from build123d import *

# Parameters (mm, degrees)
SKETCH_1_R          = 1.1
SKETCH_1_R_2        = 1.6
EXTRUDE_1_DEPTH     = 4
SKETCH_2_W          = 4
SKETCH_2_H          = 6
EXTRUDE_2_DEPTH     = 36
SKETCH_3_R          = 1.6
EXTRUDE_3_DEPTH     = 4
SKETCH_4_W          = 26
SKETCH_4_H          = 5
EXTRUDE_4_DEPTH     = 6
SKETCH_7_R          = 1.1
CUT_EXTRUDE_2_DEPTH = 66.61562314


with BuildPart() as part:
    # ｽｹｯﾁ1 → ﾎﾞｽ - 押し出し1 (new body)
    with BuildSketch(Plane.XY):
        with BuildLine():
            Line((-17, -17), (-17, -23))
            Line((-17, -23), (17, -23))
            Line((17, -23), (17, -17))
            Line((17, -17), (11, -17))
            ThreePointArc((11, -17), (8.878679656, -16.121320344), (8, -14))
            Line((8, -14), (8, 0))
            ThreePointArc((8, 0), (0, 8), (-8, 0))
            Line((-8, 0), (-8, -14))
            ThreePointArc((-8, -14), (-8.878679656, -16.121320344), (-11, -17))
            Line((-11, -17), (-17, -17))
        make_face()
        with Locations((0, 6)):
            Circle(SKETCH_1_R, mode=Mode.SUBTRACT)
        with Locations((4.242640687, 4.242640687)):
            Circle(SKETCH_1_R, mode=Mode.SUBTRACT)
        with Locations((6, 0)):
            Circle(SKETCH_1_R, mode=Mode.SUBTRACT)
        with Locations((4.242640687, -4.242640687)):
            Circle(SKETCH_1_R, mode=Mode.SUBTRACT)
        with Locations((0, -6)):
            Circle(SKETCH_1_R, mode=Mode.SUBTRACT)
        with Locations((-4.242640687, -4.242640687)):
            Circle(SKETCH_1_R, mode=Mode.SUBTRACT)
        with Locations((-6, 0)):
            Circle(SKETCH_1_R, mode=Mode.SUBTRACT)
        with Locations((-4.242640687, 4.242640687)):
            Circle(SKETCH_1_R, mode=Mode.SUBTRACT)
        Circle(SKETCH_1_R_2, mode=Mode.SUBTRACT)
    extrude(amount=EXTRUDE_1_DEPTH)

    # ｽｹｯﾁ2 → ﾎﾞｽ - 押し出し2 (add)
    with BuildSketch(Plane.XY.offset(4)):
        with Locations((-15, -20)):
            Rectangle(SKETCH_2_W, SKETCH_2_H)
        with Locations((15, -20)):
            Rectangle(SKETCH_2_W, SKETCH_2_H)
    extrude(amount=EXTRUDE_2_DEPTH)

    # ｽｹｯﾁ3 → ﾎﾞｽ - 押し出し3 (add)
    with BuildSketch(Plane.XY.offset(40)):
        with BuildLine():
            Line((-11, -17), (-17, -17))
            Line((-17, -17), (-17, -23))
            Line((-17, -23), (17, -23))
            Line((17, -23), (17, -17))
            Line((17, -17), (11, -17))
            ThreePointArc((11, -17), (8.878679656, -16.121320344), (8, -14))
            Line((8, -14), (8, 0))
            ThreePointArc((8, 0), (0, 8), (-8, 0))
            Line((-8, 0), (-8, -14))
            ThreePointArc((-8, -14), (-8.878679656, -16.121320344), (-11, -17))
        make_face()
        Circle(SKETCH_3_R, mode=Mode.SUBTRACT)
    extrude(amount=EXTRUDE_3_DEPTH)

    # ｽｹｯﾁ4 → ﾎﾞｽ - 押し出し4 (add)
    with BuildSketch(Plane(origin=(0, -17, 0), x_dir=(1, 0, 0), z_dir=(0, 1, 0))):
        with Locations((0, -6.5)):
            Rectangle(SKETCH_4_W, SKETCH_4_H)
        with Locations((0, -37.5)):
            Rectangle(SKETCH_4_W, SKETCH_4_H)
    extrude(amount=-EXTRUDE_4_DEPTH)

    # ｽｹｯﾁ7 → ｶｯﾄ - 押し出し2 (cut, through all)
    with BuildSketch(Plane(origin=(-25.9, 0, 44), x_dir=(-1, 0, 0), z_dir=(0, 0, -1))):
        with Locations((-36.4, -20)):
            Circle(SKETCH_7_R)
        with Locations(Location((-15.4, -20, 0), (0, 0, 180))):
            Circle(SKETCH_7_R)
    extrude(amount=CUT_EXTRUDE_2_DEPTH, mode=Mode.SUBTRACT)


solid = part.part
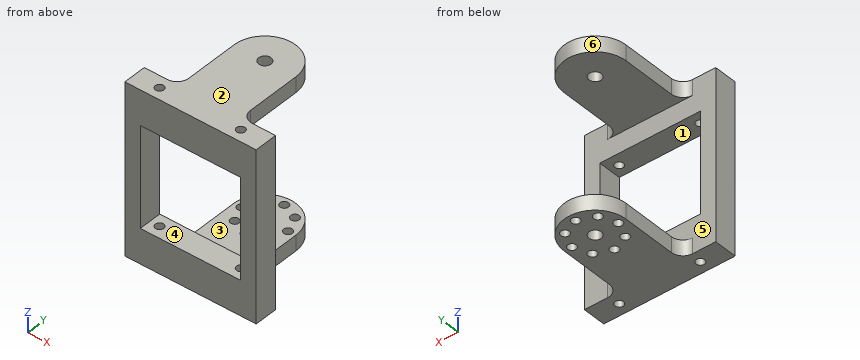
Check sheet for the modelled part. Datum: model origin and axes. Units: mm. Face numbers are marked on the shaded views. A direction names the side the tool comes from. Give positions to 0.01 mm unless a question says otherwise; leave off trailing zeros. Write each loop counter-clockwise with the first axis right and the second up, starting at its lowest first coordinate (ties: lowest second). Pieces come first, ordered by that corner, then holes. Notation, with made-up numbers: (-6.75, 49.25) -> (38.25, 49.25) arc R13 cw to (38.25, 66.25) -> close; hole circle Ø2 at (23.25, 87.5). An arc over 180 degrees is marked (long way). Write item = value, one per line.
Item 1: Sectioned sample at A-A on x = 0. Record the boundary of the cut face in (y, z).
Output:
outline = (-23, 0) -> (-7.1, 0) -> (-7.1, 4) -> (-17, 4) -> (-17, 9) -> (-23, 9) -> close; (-23, 35) -> (-17, 35) -> (-17, 40) -> (-1.6, 40) -> (-1.6, 44) -> (-23, 44) -> close; (-4.9, 0) -> (-1.6, 0) -> (-1.6, 4) -> (-4.9, 4) -> close; (1.6, 0) -> (4.9, 0) -> (4.9, 4) -> (1.6, 4) -> close; (1.6, 40) -> (8, 40) -> (8, 44) -> (1.6, 44) -> close; (7.1, 0) -> (8, 0) -> (8, 4) -> (7.1, 4) -> close
Item 2: Scan lines: probe 1 along Y at (x, z) = (0, 2.2); probe 2 along Z at (x, y) = (-6, 3); probe 3 along Z at (x, y) = (3.5, -21). Record each from-to range of solid material in increasing order. Write a range as from..to.
Output:
probe_1 = -23..-7.1, -4.9..-1.6, 1.6..4.9, 7.1..8
probe_2 = 0..4, 40..44
probe_3 = 0..9, 35..44
Item 3: Gauge pin test, flat ends, axial feed: pin 1 (10 mm diameter, centred on x = 1, z = 13.5, fed in from +Y); pin 2 (4.5 mm diameter, centred on y = -4.5, z = 42, fed in from -X). Record the tip position at first contact, or that the pin passes through.
Output:
pin_1 = -17
pin_2 = -8
Item 4: Tool access check on the marked faces 1, 2 and 3. Record the directions out of +Z, -Z, +X, -X, +Y, -Y that give a thin tool (end or side, any length) a straight path to the whole face; none if there is none.
Output:
face_1 = +Y, -Y
face_2 = +Z, +X, -X, +Y, -Y
face_3 = +X, -X, +Y
Item 5: Release check for a two-part mould opening along X. For the marked faces 4, 5 and 6 record: +X half, -X half, draft (parallel to the pull), parting line (faces both ways), or undercut.
Output:
face_4 = undercut
face_5 = draft
face_6 = parting line
Item 6: Sectioned sample at B-B on y = -20. Record the boundary of the cut face in (x, z), and give its area (3 significant figures).
Output:
outline = (-17, 0) -> (-11.6, 0) -> (-11.6, 9) -> (-13, 9) -> (-13, 35) -> (-11.6, 35) -> (-11.6, 44) -> (-17, 44) -> close; (-9.4, 0) -> (9.4, 0) -> (9.4, 9) -> (-9.4, 9) -> close; (-9.4, 35) -> (9.4, 35) -> (9.4, 44) -> (-9.4, 44) -> close; (11.6, 0) -> (17, 0) -> (17, 44) -> (11.6, 44) -> (11.6, 35) -> (13, 35) -> (13, 9) -> (11.6, 9) -> close
area = 741 mm^2
Item 7: Sectioned sample at D-D on y = -13. Record the boundary of the cut face in (x, z).
Output:
outline = (-8, 0) -> (8, 0) -> (8, 4) -> (-8, 4) -> close; (-8, 40) -> (8, 40) -> (8, 44) -> (-8, 44) -> close
Item 8: Sectioned sample at C-C on z = 11. Record the boundary of the cut face in (x, y), and give its area (3 significant figures).
Output:
outline = (-17, -23) -> (-13, -23) -> (-13, -17) -> (-17, -17) -> close; (13, -23) -> (17, -23) -> (17, -17) -> (13, -17) -> close
area = 48.0 mm^2
